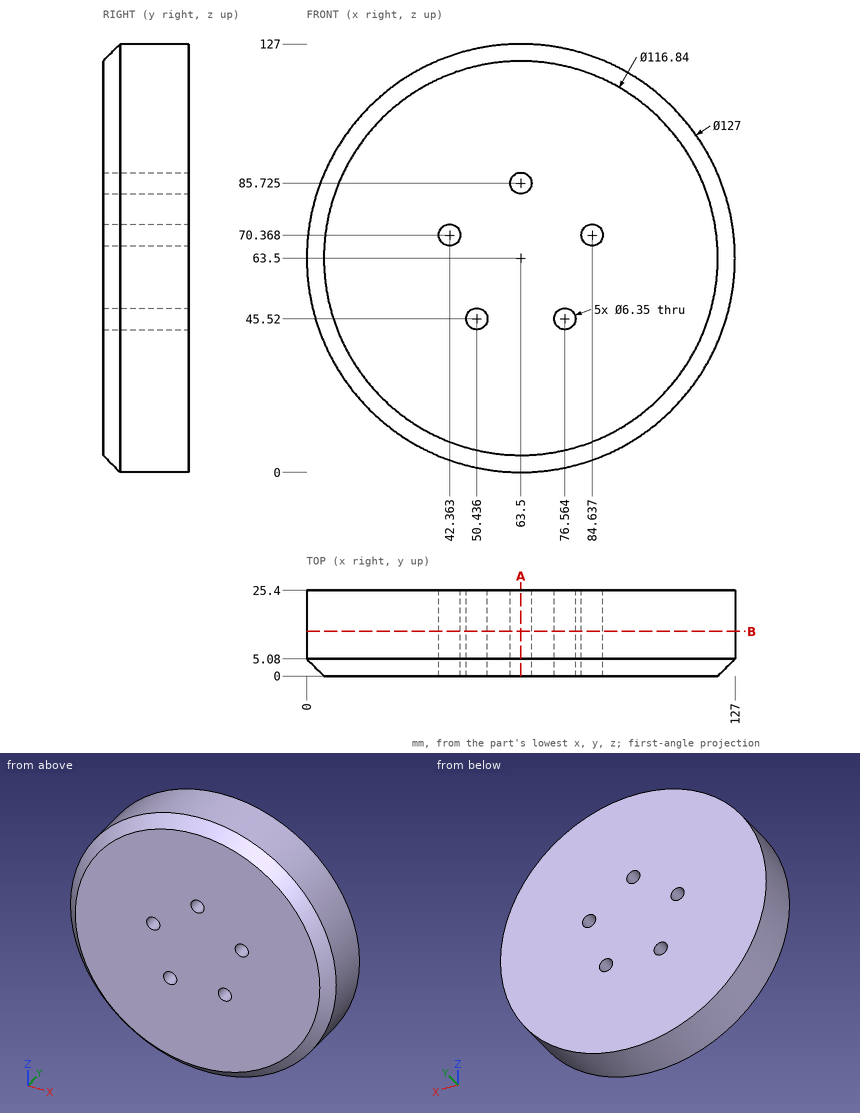
For this review, use the dimensioned drawing (mm, ordinates from the lowest corner) and the shaded views. Round coordinates to 2 decimals unless told otherwise and drop trailing zeros. Loops run counter-clockwise (first coordinate to the right, second up) from the corner with the lowest first, then second, coordinate; pieces in that order, holes last. Notation, with made-up numbers: (66.5, 77) -> (124.5, 77) arc R27 cw to (124.5, 107) -> close; hole circle Ø3 at (42, -38.5). An arc over 180 degrees is marked (long way). Write item = value, one per line. Start each with the question number.
Item 1: Take a section at A-A on x = 63.5. Give the boundary of the cut face in (y, z).
Item 2: Take a section at B-B on y = 13.25. Count the separate pieces of the cut face and the enclosed holes in it, plus the area to 3 significant figures.
Item 3: Insertion check: pin 1 (2 mm diameter, centred on y = 9, z = 50, fed in from -X); pin 2 (3 mm diameter, centred on x = 107.5, y = 20, fed in from +Z); pin 3 (6 mm diameter, centred on y = 10.5, z = 77, fed in from -X); pin 4 (7.5 mm diameter, centred on x = 76.56, z = 45.52, fed in from +Y). Each pin has a flat end and moves straight along its axis. Give the tip position at first contact, or say it passes through.
Item 4: To check wall thickness, follow L1, parallel to Z at x = 78.5, y = 7.5 (1 decimal); L2, parallel to Z at x = 62, y = 4.5 (1 decimal); L3, parallel to X at y = 23.75, z = 68.5 (1 decimal). State the ranges of each line that lie inside material, in increasing order.
Result:
q1.outline = (0, 5.08) -> (5.08, 0) -> (25.4, 0) -> (25.4, 82.55) -> (0, 82.55) -> close; (0, 88.9) -> (25.4, 88.9) -> (25.4, 127) -> (5.08, 127) -> (0, 121.92) -> close
q2.separate_pieces = 1
q2.enclosed_holes = 5
q2.area = 12,500 mm²
q3.pin_1 = 1.24
q3.pin_2 = 110.68
q3.pin_3 = 0.87
q3.pin_4 = 25.4
q4.L1 = 1.8 to 43, 48 to 125.2
q4.L2 = 0.6 to 82.9, 88.5 to 126.4
q4.L3 = 0.2 to 39.8, 44.9 to 82.1, 87.2 to 126.8
